from build123d import *

# Parameters (mm, degrees)
EXTRUDE_START   = 9
EXTRUDE_1_DEPTH = 6


with BuildPart() as part:
    # Revolve profile 1 → Revolve 1 (revolve)
    with BuildSketch(Plane(origin=(0, 0, 0), x_dir=(1, 0, 0), z_dir=(0, 1, 0)), mode=Mode.PRIVATE) as revolve_1_sk:
        Polygon((0, 0), (17, 0), (17, -5), (13, -9), (0, -9), align=None)
    revolve(revolve_1_sk.sketch.rotate(Axis((0, 0, -5), (0, 0, 1)), 180), axis=Axis((0, 0, -5), (0, 0, 1)))


with BuildPart() as body_2:
    # Extrude sketch 1 → Extrude 1 (new body)
    with BuildSketch(Plane.XY.offset(EXTRUDE_START)):
        Polygon((7, 4.041451884), (0, 8.082903769), (-7, 4.041451884), (-7, -4.041451884), (0, -8.082903769), (7, -4.041451884), align=None)
    extrude(amount=EXTRUDE_1_DEPTH)


with BuildPart() as part_1:
    add(part.part)

    # Combine _weld _ assembly of features: union body 2
    add(body_2.part)


solid = part_1.part
Could you check a few things on this model? Use its own coordinates, in mm. A direction names the side the tool comes from. Coordinates: 2 decimals unless noted, no trailing zeros. Write each loop counter-clockwise with the first axis right and the second up, starting at its lowest first coordinate (ties: lowest second). Pieces come first, ordered by that corner, then holes. Notation, with made-up numbers: (68.25, 43) - (125.25, 43) arc R15 cw to (125.25, 66) - close; hole circle Ø6 at (64, 26.5). An arc over 180 degrees is marked (long way). Put each result on its own line as item: value. Start each with the question number.
Q1. I'm going to push flat-ended pins straight in: P1, Ø3, axis at y = -1.5, z = 12, coming from the -X side; P2, Ø4, axis at x = 2, y = -11, coming from the +Z side; P3, Ø4, axis at y = -7, z = 8.5, coming from the +X side. Where does each tip first touch, or does it pass through?
Q2. Please list where these lines run through material, in increasing order: L1, parallel to Z at x = 11, y = -4.5; L2, parallel to X at y = 5.5, z = 11; L3, parallel to X at y = 10.5, z = 5.5.
Q3. Which directions (+Z, -Z, +X, -X, +Y, -Y) give clear straight access to the entire face, cutting with the end or side of a thin tool? Please do faces 1 (the flat face through (7, 0, 12)), 2 (the flat face through (3.45, -6.09, 11.96)), 3 (the flat face through (-7, 0, 12)), 4 (the flat face through (3.549, 6.034, 11.958)).
Q4. I want a section at B-B on z = 11.5. Write out the boundary of the cut face in (x, y).
Q5. I want a section at C-C on z = 6. Write out the boundary of the cut face in (x, y), plus the area to 3 significant figures.
Q6. I want a section at A-A on y = 0. Write out the boundary of the cut face in (x, z), plus the area to 3 significant figures.
Checks:
1. P1: x = -7
1. P2: z = 9
1. P3: x = 14.02
2. L1: 0 to 9
2. L2: -4.47 to 4.47
2. L3: -12.73 to 12.73
3. face 1: +Z, +X, +Y, -Y
3. face 2: +Z, +X, -Y
3. face 3: +Z, -X, +Y, -Y
3. face 4: +Z, +X, +Y
4. outline: (-7, -4.04) - (0, -8.08) - (7, -4.04) - (7, 4.04) - (0, 8.08) - (-7, 4.04) - close
5. outline: circle Ø32 at (0, 0)
5. area: 804 mm²
6. outline: (-17, 0) - (17, 0) - (17, 5) - (13, 9) - (7, 9) - (7, 15) - (-7, 15) - (-7, 9) - (-13, 9) - (-17, 5) - close
6. area: 374 mm²
